from build123d import *

# Parameters (mm, degrees)
BOSS_EXTRUDE1_DEPTH      = 19.09
BOSS_EXTRUDE1_DEPTH_BACK = 19.09
CUT_EXTRUDE1_DEPTH       = 7.36
SKETCH3_R                = 1.125
CUT_EXTRUDE2_DEPTH       = 6.35
SKETCH4_R                = 1.65
CUT_EXTRUDE3_DEPTH       = 15


with BuildPart() as part:
    # Sketch1 → Boss-Extrude1 (new body, two sides)
    with BuildSketch(Plane.XY) as boss_extrude1_sk:
        Polygon((-3.18, 0), (3.18, 0), (3.18, 10.34), (17.43, 10.34), (17.43, 19.87), (-3.18, 19.87), align=None)
    extrude(amount=BOSS_EXTRUDE1_DEPTH)
    extrude(boss_extrude1_sk.sketch, amount=-BOSS_EXTRUDE1_DEPTH_BACK)

    # Sketch2 → Cut-Extrude1 (cut, through all)
    with BuildSketch(Plane(origin=(3.18, 0, 0), x_dir=(0, 0, -1), z_dir=(1, 0, 0))):
        Polygon((19.09, 10.34), (6.31, 0), (19.09, 0), align=None)
        Polygon((-19.09, 10.34), (-19.09, 0), (-6.31, 0), align=None)
    extrude(amount=-CUT_EXTRUDE1_DEPTH, mode=Mode.SUBTRACT)

    # Sketch3 → Cut-Extrude2 (cut)
    with BuildSketch(Plane.XZ):
        Circle(SKETCH3_R)
    extrude(amount=-CUT_EXTRUDE2_DEPTH, mode=Mode.SUBTRACT)

    # Sketch4 → Cut-Extrude3 (cut)
    with BuildSketch(Plane(origin=(17.43, 0, 0), x_dir=(0, 0, -1), z_dir=(1, 0, 0))):
        with Locations((9.53, 15.045)):
            Circle(SKETCH4_R)
        with Locations((-9.53, 15.045)):
            Circle(SKETCH4_R)
    extrude(amount=-CUT_EXTRUDE3_DEPTH, mode=Mode.SUBTRACT)


solid = part.part
Model file for the job. Use its own axes, mm. A direction names the side the tool comes from. Give positions to 0.01 mm unless a question says otherwise; leave off trailing zeros. Write each loop counter-clockwise with the first axis right and the second up, starting at its lowest first coordinate (ties: lowest second). Pieces come first, ordered by that corner, then holes. Notation, with made-up numbers: M 14.5,58 L 21.5,58 A27 ccw 21.5,74 Z; hole C 30.5,54.25 d2. An arc over 180 degrees is marked long. One line per item, written item: value. Start each with the question number.
Q1. Drop flat-ended pins along their axis: pin 1 Ø2 at (x, z) = (9.5, -15) entering from -Y; pin 2 Ø1.7 at (y, z) = (14.5, -9.5) entering from +X; pin 3 Ø0.7 at (x, z) = (-0.5, -0.5) entering from -Y. Give the stop position or say it passes through.
Q2. Saw through at A-A, the plane x = 0. Write the cut outline in (y, z) (3 decimals).
Q3. Saw through at D-D, the plane x = 10.5. Write the cut outline in (y, z) (3 decimals).
Q4. 3-axis set-ups, long thin cutter, end or side, ignore diameter. For faces 4 (the flat face through (7, 19.87, 0)), 5 (the flat face through (-3.18, 12, 0)), 6 (the cylindrical face through (-0.146, 3.131, 1.115)), 7 (the flat face through (10, 10.34, 0)), 8 (the flat face through (2.43, 15, 10)): which of +Z, -Z, +X, -X, +Y, -Y reach the whole face in a straight line?
Q5. Two-plate mould, pull along X, no slides. Class faces 1 (the flat face through (7, 15, 19.09)), 2 (the flat face through (0, 6.35, 0)), 3 (the flat face through (3.18, 6, 0)): +X half, -X half, draft (parallel to the pull), parting line (faces both ways), or undercut.
Q6. Saw through at C-C, the plane y = 15.5. Write the cut outline in (x, z), plus the area to 3 significant figures.
Q7. Saw through at B-B, the plane z = -5. Write the cut outline in (x, y), plus the area to 3 significant figures.
Q8. Probe probe 1 along Y at (x, z) = (8.25, -9.53) (3 decimals); probe 2 along Y at (x, z) = (13, 6.5); probe 3 along X at (y, z) = (9.5, 12). List the from-to ranges inside material, lowest first. Write a range as [from, to].
Output values:
1. pin 1: stops at y = 10.34
1. pin 2: stops at x = 2.43
1. pin 3: stops at y = 6.35
2. outline: M 0,-6.31 L 10.34,-19.09 L 19.87,-19.09 L 19.87,19.09 L 10.34,19.09 L 0,6.31 L 0,1.125 L 6.35,1.125 L 6.35,-1.125 L 0,-1.125 Z
3. outline: M 10.34,-19.09 L 19.87,-19.09 L 19.87,19.09 L 10.34,19.09 Z; hole C 15.045,-9.53 d3.3; hole C 15.045,9.53 d3.3
4. face 4: +Z, -Z, +X, -X, +Y
4. face 5: +Z, -Z, -X, +Y, -Y
4. face 6: -Y
4. face 7: +Z, -Z, +X, -Y
4. face 8: +X
5. face 1: draft
5. face 2: undercut
5. face 3: +X half
6. outline: M -3.18,-19.09 L 17.43,-19.09 L 17.43,-11.12 L 2.43,-11.12 L 2.43,-7.94 L 17.43,-7.94 L 17.43,7.94 L 2.43,7.94 L 2.43,11.12 L 17.43,11.12 L 17.43,19.09 L -3.18,19.09 Z
6. area: 692 mm²
7. outline: M -3.18,0 L 3.18,0 L 3.18,10.34 L 17.43,10.34 L 17.43,19.87 L -3.18,19.87 Z
7. area: 262 mm²
8. probe 1: y = [10.34, 13.395], [16.695, 19.87]
8. probe 2: y = [10.34, 19.87]
8. probe 3: x = [-3.18, 3.18]
